from build123d import *

# Parameters (mm, degrees)
SKICA5_W                 = 12.05
SKICA5_H                 = 10.05
P_IDAT_VYSUNUT_M5_DEPTH  = 0.8
ZAOBLIT2_R               = 1
SKICA6_R                 = 1.5
P_IDAT_VYSUNUT_M6_DEPTH  = 7.4
LINPOLE1_COUNT           = 2
LINPOLE1_PITCH           = 3.1
ZAOBLIT2_OF_LINPOLE1_R   = 1
LINPOLE2_COUNT           = 2
LINPOLE2_PITCH           = 8.2
ZAOBLIT2_OF_LINPOLE2_R   = 1
SKICA7_R                 = 2
SKICA7_R_2               = 1.015
P_IDAT_VYSUNUT_M7_DEPTH  = 0.8
SKICA9_R                 = 1.015
ODEBRAT_VYSUNUT_M2_DEPTH = 10.8


with BuildPart() as part:
    # Skica5 → Přidat vysunutím5 (new body)
    with BuildSketch(Plane.XY):
        Rectangle(SKICA5_W, SKICA5_H)
    p_idat_vysunut_m5 = extrude(amount=P_IDAT_VYSUNUT_M5_DEPTH)

    # Zaoblit2
    zaoblit2_edges = [part.edges().sort_by_distance(p)[0] for p in [
        (6.025, -5.025, 0.4),
        (-6.025, -5.025, 0.4),
        (-6.025, 5.025, 0.4),
        (6.025, 5.025, 0.4),
    ]]
    fillet(zaoblit2_edges, radius=ZAOBLIT2_R)

    # Skica6 → Přidat vysunutím6 (add)
    with BuildSketch(Plane.XY.offset(0.8)):
        with Locations((3.625, 2.625)):
            Circle(SKICA6_R)
        with Locations((-3.625, -2.625)):
            Circle(SKICA6_R)
    extrude(amount=P_IDAT_VYSUNUT_M6_DEPTH)

    # LinPole1: Přidat vysunutím5 ×2
    with Locations(*[(0, 0, i * LINPOLE1_PITCH) for i in range(1, LINPOLE1_COUNT)]):
        add(p_idat_vysunut_m5)

    # Zaoblit2 of LinPole1
    zaoblit2_of_linpole1_edges = [part.edges().sort_by_distance(p)[0] for p in [
        (6.025, -5.025, 3.5),
        (-6.025, -5.025, 3.5),
        (-6.025, 5.025, 3.5),
        (6.025, 5.025, 3.5),
    ]]
    fillet(zaoblit2_of_linpole1_edges, radius=ZAOBLIT2_OF_LINPOLE1_R)

    # LinPole2: Přidat vysunutím5 ×2
    with Locations(*[(0, 0, i * LINPOLE2_PITCH) for i in range(1, LINPOLE2_COUNT)]):
        add(p_idat_vysunut_m5)

    # Zaoblit2 of LinPole2
    zaoblit2_of_linpole2_edges = [part.edges().sort_by_distance(p)[0] for p in [
        (6.025, -5.025, 8.6),
        (-6.025, -5.025, 8.6),
        (-6.025, 5.025, 8.6),
        (6.025, 5.025, 8.6),
    ]]
    fillet(zaoblit2_of_linpole2_edges, radius=ZAOBLIT2_OF_LINPOLE2_R)

    # Skica7 → Přidat vysunutím7 (add)
    with BuildSketch(Plane.XY.offset(9)):
        Circle(SKICA7_R)
        Circle(SKICA7_R_2, mode=Mode.SUBTRACT)
    extrude(amount=P_IDAT_VYSUNUT_M7_DEPTH)

    # Skica9 → Odebrat vysunutím2 (cut, through all)
    with BuildSketch(Plane.XY):
        Circle(SKICA9_R)
    extrude(amount=ODEBRAT_VYSUNUT_M2_DEPTH, mode=Mode.SUBTRACT)


solid = part.part
Could you check a few things on this model? Use its own coordinates, in mm. A direction names the side the tool comes from. Give positions to 0.01 mm unless a question says otherwise; leave off trailing zeros. Order: outer loops, then holes, each group sorted by start corner. A loop starts at its lowest first (then second) coordinate and runs counter-clockwise, first axis right, second up. Notation, with made-up numbers: (52.25, 81.5) - (58.25, 81.5) arc R14 cw to (58.25, 95.5) - close; hole circle Ø8 at (-16.5, 87). An arc over 180 degrees is marked (long way). One line per item, written item: value. Start each with the question number.
1. Imagine slicing it at A-A on y = 0. List the corners of the cut face in (x, z) for me (3 decimals), plus the area to 3 significant figures.
2. If I drill on probe 1 along Z at (x, y) = (5, -3.75); probe 2 along Z at (x, y) = (-0.5, -1.5); probe 3 along X at (y, z) = (0, 0.3) (3 decimals), over which ranges is the centre line in solid material (lowest first)?
3. For faces 4 (the face through (-0.1, 1.2, 0.8)), 5 (the face through (-0.1, 2.3, 9)), 6 (the face through (0.546, 0.856, 3.494)), which set-ups out of +Z, -Z, +X, -X, +Y, -Y let a thin tool reach every point of the face, with its end or its side?
4. Imagine slicing it at D-D on y = -2.25. List the corners of the cut face in (x, z) for me (3 decimals).
5. For P1, Ø2.5, axis at x = 0, y = 0, coming from the -Z side; P2, Ø1.5, axis at x = -3.5, z = 7, coming from the -Y side (3 decimals), each with a flat end and sliding along its axis, tell me the tip position at first contact or that it passes through.
6. Imagine slicing it at C-C on x = 5.5. List the corners of the cut face in (y, z) for me.
7. Imagine slicing it at B-B on x = 0. List the corners of the cut face in (y, z) for me (3 decimals).
8. Thinking about a two-plate mould opening in Y: for faces 1 (the face through (-2.194, -2.174, 6.02)), 2 (the face through (0.546, 0.856, 0.394)), 3 (the face through (-0.1, 1.2, 8.2)), which applies, +Y half, -Y half, draft (parallel to the pull), parting line (faces both ways), or undercut?
Values:
1. outline: (-6.025, 0) - (-1.015, 0) - (-1.015, 0.8) - (-6.025, 0.8) - close; (-6.025, 3.1) - (-1.015, 3.1) - (-1.015, 3.9) - (-6.025, 3.9) - close; (-6.025, 8.2) - (-1.015, 8.2) - (-1.015, 9.8) - (-2, 9.8) - (-2, 9) - (-6.025, 9) - close; (1.015, 0) - (6.025, 0) - (6.025, 0.8) - (1.015, 0.8) - close; (1.015, 3.1) - (6.025, 3.1) - (6.025, 3.9) - (1.015, 3.9) - close; (1.015, 8.2) - (6.025, 8.2) - (6.025, 9) - (2, 9) - (2, 9.8) - (1.015, 9.8) - close
1. area: 25.6 mm²
2. probe 1: 0 to 0.8, 3.1 to 3.9, 8.2 to 9
2. probe 2: 0 to 0.8, 3.1 to 3.9, 8.2 to 9.8
2. probe 3: -6.025 to -1.015, 1.015 to 6.025
3. face 4: none
3. face 5: +Z
3. face 6: +Z, -Z
4. outline: (-6.025, 0) - (6.025, 0) - (6.025, 0.8) - (-2.173, 0.8) - (-2.173, 3.1) - (6.025, 3.1) - (6.025, 3.9) - (-2.173, 3.9) - (-2.173, 8.2) - (6.025, 8.2) - (6.025, 9) - (-6.025, 9) - (-6.025, 8.2) - (-5.077, 8.2) - (-5.077, 3.9) - (-6.025, 3.9) - (-6.025, 3.1) - (-5.077, 3.1) - (-5.077, 0.8) - (-6.025, 0.8) - close
5. P1: z = 0
5. P2: y = -4.125
6. outline: (-4.9, 0) - (4.9, 0) - (4.9, 0.8) - (-4.9, 0.8) - close; (-4.9, 3.1) - (4.9, 3.1) - (4.9, 3.9) - (-4.9, 3.9) - close; (-4.9, 8.2) - (4.9, 8.2) - (4.9, 9) - (-4.9, 9) - close
7. outline: (-5.025, 0) - (-1.015, 0) - (-1.015, 0.8) - (-5.025, 0.8) - close; (-5.025, 3.1) - (-1.015, 3.1) - (-1.015, 3.9) - (-5.025, 3.9) - close; (-5.025, 8.2) - (-1.015, 8.2) - (-1.015, 9.8) - (-2, 9.8) - (-2, 9) - (-5.025, 9) - close; (1.015, 0) - (5.025, 0) - (5.025, 0.8) - (1.015, 0.8) - close; (1.015, 3.1) - (5.025, 3.1) - (5.025, 3.9) - (1.015, 3.9) - close; (1.015, 8.2) - (5.025, 8.2) - (5.025, 9) - (2, 9) - (2, 9.8) - (1.015, 9.8) - close
8. face 1: parting line
8. face 2: undercut
8. face 3: draft
